Check sheet for the modelled part. Datum: model origin and axes. Units: mm. A direction names the side the tool comes from. Round coordinates to 2 decimals unless told otherwise and drop trailing zeros. Loops run counter-clockwise (first coordinate to the right, second up) from the corner with the lowest first, then second, coordinate; pieces in that order, holes last. Notation, with made-up numbers: (29.5, 2) - (68.5, 2) arc R31 cw to (68.5, 28) - close; hole circle Ø3 at (28.5, 67.5). An arc over 180 degrees is marked (long way). Answer in a Markdown table with one row per item. Add a question column.
(1) Mould release check, pull along X, two halves, no side actions. Record for faces 3 (the flat face through (-27.151, 17, 7)), 4 (the flat face through (-26.08, -27.07, 7.1)), 5 (the flat face through (-18, 11, 0)), 6 (the cylindrical face through (-28.27, -12.2, 6.9)): +X half, -X half, draft (parallel to the pull), parting line (faces both ways), or undercut.
(2) Gauge pin test, flat ends, axial feed: pin 1 (1 mm diameter, centred on x = -14, z = 9.5, fed in from +Y); pin 2 (7 mm diameter, centred on x = -13.2, y = 17.24, fed in from +Z); pin 3 (4 mm diameter, centred on y = 16.5, z = 5.5, fed in from -X); pin 4 (3 mm diameter, centred on x = -33.5, z = 6.5, fed in from +Y). Record the tip position at first contact, or that the pin passes through.
(3) Thickness scan on line 1 along Y through (x, z) = (-13.2, 7); line 2 along Y through (x, z) = (-19, 10); line 3 along Y through (x, z) = (-11, 7.5). Record the ranges inside material, lowest first.
(4) Cross-section at C-C on x = -35.5. Enter the section's corners in (y, z), then the cut area to 3 significant figures.
(5) Cross-section at A-A on z = 7.25. Enter the section's corners in (x, y), then the cut area to 3 significant figures.
(6) Access from +Z, -Z, +X, -X, +Y, -Y to the whole of each face (thin tool, end or side, straight path). Record for faces 1 (the flat face through (-36.402, -21.108, 6.902)), 2 (the flat face through (0, 17, 7)).
(7) Cross-section at D-D on x = -24.5. Count the separate pieces of the cut face and the enclosed holes in it, then the cut area to 3 significant figures.
(8) Cross-section at B-B on y = 17.24. Enter the section's corners in (x, z).
Autodesk Inventor part; units mm, degrees
ref_plane "YZ Plane" through (0, 0, 0) normal (1, 0, 0) x (0, 1, 0)
ref_plane "XZ Plane" through (0, 0, 0) normal (0, 1, 0) x (-1, 0, 0)
ref_plane "XY Plane" through (0, 0, 0) normal (0, 0, 1) x (1, 0, 0)
sketch "Sketch1" plane through (0, 0, 0) normal (0, 0, 1) x (1, 0, 0)
  line L0 (0, 0) -> (0, 34.48)
  line L1 (0, 34.48) -> (-11.25, 53.9656)
  line L2 (-11.25, 53.9656) -> (-23.6139, 57.2785)
  line L3 (-23.6139, 57.2785) -> (-33.9369, 51.3185)
  line L4 (-33.9369, 51.3185) -> (-37.2963, 38.7807)
  line L5 (-37.2963, 38.7807) -> (-27.1513, 21.2091)
  line L6 (-37.2963, -4.3007) -> (-33.9369, -16.8385)
  line L7 (-33.9369, -16.8385) -> (-23.6139, -22.7985)
  line L8 (-23.6139, -22.7985) -> (-11.25, -19.4856)
  line L9 (-11.25, -19.4856) -> (0, 0)
  line L10 (-37.2963, -4.3007) -> (-27.1513, 13.2709)
  line L11 (-27.1513, 13.2709) -> (-27.1513, 21.2091)
  circle A0 centre (-24.2754, 46.5042) radius 4
  circle A1 centre (-24.2754, -12.0242) radius 4
  line L12 (-33.9369, -16.8385) -> (-57.9984, -2.9465)
  line L13 (-33.9369, -16.8385) -> (-24.2152, 0)
  line L14 (-27.1513, 55.2361) -> (-5.625, 67.6643)
  line L15 (-23.6139, 57.2785) -> (-11.8125, 36.8379)
  circle A2 centre (-13.2, 17.24) radius 4
  dimension "d0" = 34.48
  dimension "d1" = 22.5
  dimension "d2" = 12.8
  dimension "d3" = 11.92
  dimension "d4" = 12.98
  dimension "d10" = 150
  dimension "d11" = 135
  dimension "d12" = 135
  dimension "d13" = 135
  dimension "d14" = 135
  dimension "d21" = 150
  dimension "d22" = 22.5
  dimension "d23" = 135
  dimension "d24" = 12.8
  dimension "d25" = 225
  dimension "d26" = 11.92
  dimension "d27" = 12.98
  dimension "d28" = 135
  dimension "d29" = 20.29
  dimension "d30" = 135
  dimension "d31" = 7.9382
  dimension "d32" = 9
  dimension "d33" = 9
  dimension "d34" = 5.96
  dimension "d35" = 5.96
  dimension "d36" = 8
  dimension "d37" = 8
  dimension "d38" = 13.2
  dimension "d39" = 8
extrude "Extrusion1" add sketch "Sketch1" along normal blind 14
sketch "Sketch2" plane through (0, 34.48, 14) normal (0.866, 0.5, 0) x (0, 0, -1)
  line L0 (0, 22.5) -> (0, 0)
  line L1 (14, 0) -> (0, 0)
  line L2 (14, 22.5) -> (0, 22.5)
  circle A0 centre (7, 11.25) radius 4
  point P0 (14, -29.8606)
  dimension "d42" = 22.5
  dimension "d43" = 11.25
  dimension "d44" = 7
  dimension "d52" = 8
extrude "Extrusion2" cut sketch "Sketch2" against normal blind 40
sketch "Sketch3" plane through (-11.25, -19.4856, 14) normal (0.866, -0.5, 0) x (0, 0, -1)
  line L0 (14, 0) -> (14, 22.5)
  line L1 (14, 22.5) -> (0, 22.5)
  circle A0 centre (7, 11.25) radius 4
  line L2 (14, -9.051) -> (0, -9.051)
  dimension "d47" = 8
  dimension "d48" = 11.25
  dimension "d49" = 7
  dimension "d64" = 20.301
extrude "Extrusion3" cut sketch "Sketch3" against normal blind 40
sketch "Sketch5" plane through (-33.9369, -16.8385, 0) normal (-0.5, -0.866, 0) x (0.866, -0.5, 0)
  line L0 (11.92, 0) -> (0, 0)
  line L1 (0, 0) -> (0, 14)
  line L2 (0, 14) -> (11.92, 14)
  line L3 (11.92, 14) -> (11.92, 0)
  point P0 (20.971, 0)
extrude "Extrusion4" add sketch "Sketch5" along normal blind 10
properties part number "Vertex Bootm with foot"
Answers:
| question | item | result |
|---|---|---|
| 1 | face 3 | -X half |
| 1 | face 4 | +X half |
| 1 | face 5 | draft |
| 1 | face 6 | undercut |
| 2 | pin 1 | stops at y = 54.84 |
| 2 | pin 2 | passes through |
| 2 | pin 3 | stops at x = -27.15 |
| 2 | pin 4 | stops at y = 52.44 |
| 3 | line 1 | y = -20.01 to -9.99, -0.75 to 13.24, 21.24 to 35.23, 44.47 to 54.49 |
| 3 | line 2 | y = -21.56 to -5.08, 1.03 to 33.45, 39.56 to 56.04 |
| 3 | line 3 | y = -19.05 to -11.22, -2.06 to 13.9, 20.58 to 36.54, 45.7 to 53.53 |
| 4 | outline | (-27.48, 0) - (-19.55, 0) - (-19.55, 14) - (-27.48, 14) - close; (-11, 0) - (-1.19, 0) - (-1.19, 14) - (-11, 14) - close; (35.67, 0) - (45.48, 0) - (45.48, 14) - (35.67, 14) - close |
| 4 | area | 386 mm^2 |
| 5 | outline | (-38.94, -25.5) - (-28.61, -31.46) - (-23.61, -22.8) - (-11.25, -19.49) - (-7.62, -13.2) - (-33.73, 1.87) - (-37.3, -4.3) - (-33.94, -16.84) - close; (-37.3, 38.78) - (-33.73, 32.61) - (-7.62, 47.68) - (-11.25, 53.97) - (-23.61, 57.28) - (-33.94, 51.32) - close; (-29.74, 8.79) - (-3.63, -6.29) - (0, 0) - (0, 34.48) - (-3.63, 40.77) - (-29.74, 25.69) - (-27.15, 21.21) - (-27.15, 13.27) - close; hole circle Ø8 at (-24.28, -12.02); hole circle Ø8 at (-24.28, 46.5); hole circle Ø8 at (-13.2, 17.24) |
| 5 | area | 1,740 mm^2 |
| 6 | face 1 | +Z, -Z, -X |
| 6 | face 2 | +Z, -Z, +X, +Y, -Y |
| 7 | separate pieces | 3 |
| 7 | enclosed holes | 2 |
| 7 | area | 796 mm^2 |
| 8 | outline | (-27.15, 0) - (-17.2, 0) - (-17.2, 14) - (-27.15, 14) - close; (-9.2, 0) - (0, 0) - (0, 14) - (-9.2, 14) - close |
